Drawing for the job (mm, zero at the part's lowest x, y, z). Round coordinates to 2 decimals unless told otherwise and drop trailing zeros. Write each loop counter-clockwise with the first axis right and the second up, starting at its lowest first coordinate (ties: lowest second). Pieces come first, ordered by that corner, then holes.
Item 1: Drop a flat-ended pin along its axis: pin 1 Ø4 at (y, z) = (7.5, 17.5) entering from -X. Give the stop position or say it passes through.
Item 2: Band-saw the part on B-B, the plane y = 7.5. Write the cut outline in (x, z), then the cut area to 3 significant figures.
Item 3: Band-saw the part on A-A, the plane z = 17.5. Write the cut outline in (x, y), then the cut area to 3 significant figures.
Item 4: Band-saw the part on C-C, the plane x = 0.35. Write the cut outline in (y, z).
Item 5: Wall check: probe 1 along Z at (x, y) = (0.8, 7.5); probe 2 along Z at (x, y) = (2.75, 6.5); probe 3 along Y at (x, z) = (1.45, 18.5). Give the ranges that are in metal, low to high.
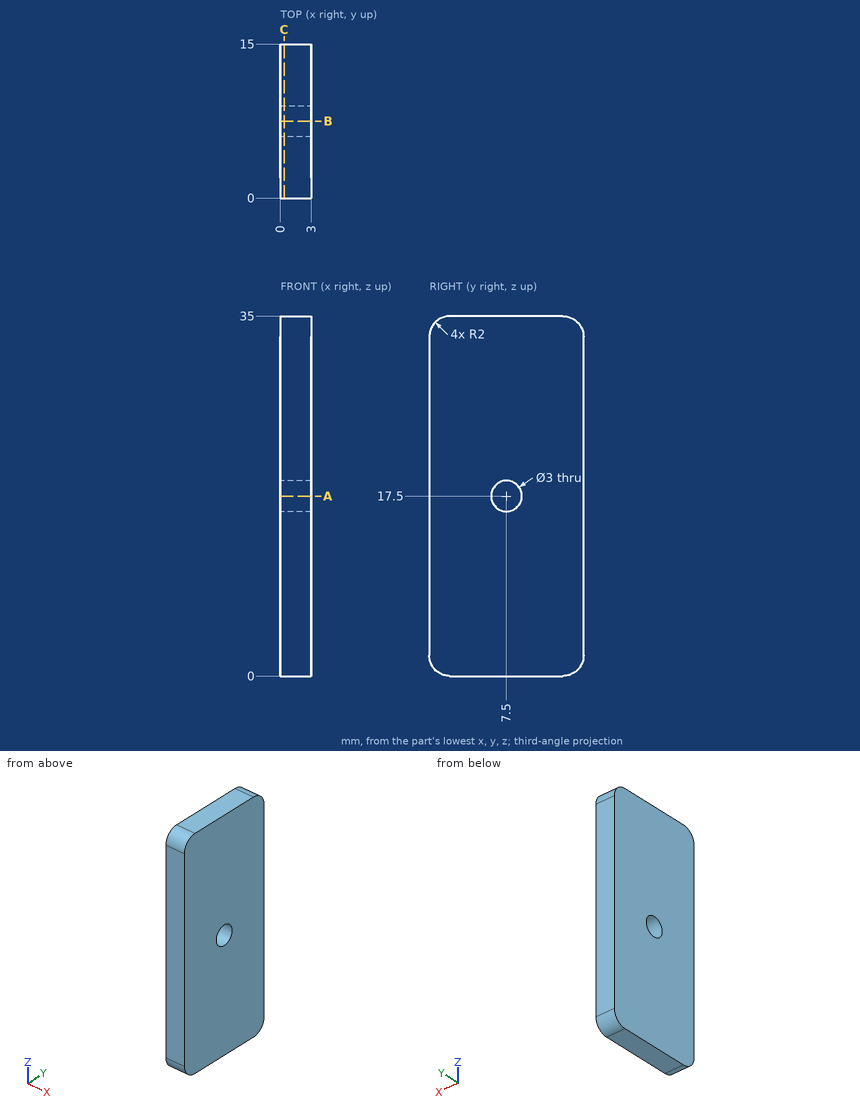
Results:
1. pin 1: stops at x = 0
2. outline: (0, 0) - (3, 0) - (3, 16) - (0, 16) - close; (0, 19) - (3, 19) - (3, 35) - (0, 35) - close
2. area: 96.0 mm2
3. outline: (0, 0) - (3, 0) - (3, 6) - (0, 6) - close; (0, 9) - (3, 9) - (3, 15) - (0, 15) - close
3. area: 36.0 mm2
4. outline: (0, 2) arc R2 ccw to (2, 0) - (13, 0) arc R2 ccw to (15, 2) - (15, 33) arc R2 ccw to (13, 35) - (2, 35) arc R2 ccw to (0, 33) - close; hole circle Ø3 at (7.5, 17.5)
5. probe 1: z = 0 to 16, 19 to 35
5. probe 2: z = 0 to 16.38, 18.62 to 35
5. probe 3: y = 0 to 6.38, 8.62 to 15
